Source: CAD feature listing. Evaluate the final solid. Frame: model axes, mm. Give positions to 0.01 mm unless a question says otherwise; leave off trailing zeros. Loops run counter-clockwise (first coordinate to the right, second up) from the corner with the lowest first, then second, coordinate; pieces in that order, holes last. Notation, with made-up numbers: (-27, 24.5) -> (-19, 24.5) arc R21 cw to (-19, 60.5) -> close; hole circle Ø10 at (37, 25.25). An arc over 180 degrees is marked (long way). Return JSON: item names as keys, results as strings. Group by question number.
(1) Ray query, line 1 (X direction, y = 2.6, z = -51.5); line 2 (Z direction, x = 35.75, y = 1.15) (3 decimals); line 3 (Z direction, x = -70.17, y = 1.1). Return the intervals inside material, ascending. Write a range as from..to.
(2) Cut plane B-B on x = -23. Return loops of the section in (y, z), then the cut area to 3 significant figures.
(3) Pin query (flat end, axial travel): pin 1 (2.5 mm diameter, centred on x = 82.67, z = -74.19, fed in from +Y). Return the tip coordinate at first contact, or that it passes through.
(4) Cut plane C-C on y = 2.4. Give the number of separate pieces and of enclosed holes in the cut face, then the cut area to 3 significant figures.
(5) Cut plane A-A on z = 33. Return loops of the section in (x, y), then the cut area to 3 significant figures.
```python
from build123d import *

# Parameters (mm, degrees)
SCHIZZO1_W                   = 180.34
SCHIZZO1_H                   = 227.22
ESTRUSIONE_ESTRUSIONE1_DEPTH = 3
SCHIZZO2_R                   = 1.5
SCHIZZO2_R_2                 = 3.25
SCHIZZO2_W                   = 5
SCHIZZO2_H                   = 18
TAGLIO_ESTRUSIONE1_DEPTH     = 4
SCHIZZO3_R                   = 1.5
TAGLIO_ESTRUSIONE5_DEPTH     = 4


with BuildPart() as part:
    # Schizzo1 → Estrusione-Estrusione1 (new body)
    with BuildSketch(Plane(origin=(0, 0, 0), x_dir=(1, 0, 0), z_dir=(0, 1, 0))):
        Rectangle(SCHIZZO1_W, SCHIZZO1_H)
    extrude(amount=ESTRUSIONE_ESTRUSIONE1_DEPTH)

    # Schizzo2 → Taglio-Estrusione1 (cut, through all)
    with BuildSketch(Plane(origin=(0, 0, 0), x_dir=(1, 0, 0), z_dir=(0, 1, 0))):
        with Locations((-82.67, -5.81)):
            Circle(SCHIZZO2_R)
        with Locations((-82.67, -87.31)):
            Circle(SCHIZZO2_R)
        with Locations((-82.67, 74.19)):
            Circle(SCHIZZO2_R)
        with Locations((82.67, -87.31)):
            Circle(SCHIZZO2_R)
        with Locations((82.67, -5.81)):
            Circle(SCHIZZO2_R)
        with Locations((82.67, 74.19)):
            Circle(SCHIZZO2_R)
        with Locations((-70.17, -78.61)):
            Circle(SCHIZZO2_R_2)
        with Locations((70.17, -78.61)):
            Circle(SCHIZZO2_R_2)
        with Locations((-30, 89.61)):
            Circle(SCHIZZO2_R)
        with Locations((-30, 108.61)):
            Circle(SCHIZZO2_R)
        with Locations((30, 89.61)):
            Circle(SCHIZZO2_R)
        with Locations((30, 108.61)):
            Circle(SCHIZZO2_R)
        with Locations((82.67, -49.13)):
            Rectangle(SCHIZZO2_W, SCHIZZO2_H)
        with Locations((-82.67, -49.13)):
            Rectangle(SCHIZZO2_W, SCHIZZO2_H)
        with Locations((-82.67, 47.19)):
            Rectangle(SCHIZZO2_W, SCHIZZO2_H)
        with Locations((82.67, 47.19)):
            Rectangle(SCHIZZO2_W, SCHIZZO2_H)
    extrude(amount=TAGLIO_ESTRUSIONE1_DEPTH, mode=Mode.SUBTRACT)

    # Schizzo3 → Taglio-Estrusione5 (cut, through all)
    with BuildSketch(Plane(origin=(0, 0, 0), x_dir=(1, 0, 0), z_dir=(0, 1, 0))):
        with Locations((-35.75, -77.045)):
            Circle(SCHIZZO3_R)
        with Locations((35.75, -77.045)):
            Circle(SCHIZZO3_R)
        with Locations((-35.75, 16.055)):
            Circle(SCHIZZO3_R)
        with Locations((35.75, 16.055)):
            Circle(SCHIZZO3_R)
        with BuildLine():
            Line((-31.5, -84.26), (-31.5, 23.27))
            ThreePointArc((-31.5, 23.27), (-30.225914498, 26.345914498), (-27.15, 27.62))
            Line((-27.15, 27.62), (27.15, 27.62))
            ThreePointArc((27.15, 27.62), (30.225914498, 26.345914498), (31.5, 23.27))
            Line((31.5, 23.27), (31.5, -84.26))
            ThreePointArc((31.5, -84.26), (30.225914498, -87.335914498), (27.15, -88.61))
            Line((27.15, -88.61), (-27.15, -88.61))
            ThreePointArc((-27.15, -88.61), (-30.225914498, -87.335914498), (-31.5, -84.26))
        make_face()
    extrude(amount=TAGLIO_ESTRUSIONE5_DEPTH, mode=Mode.SUBTRACT)


solid = part.part
```
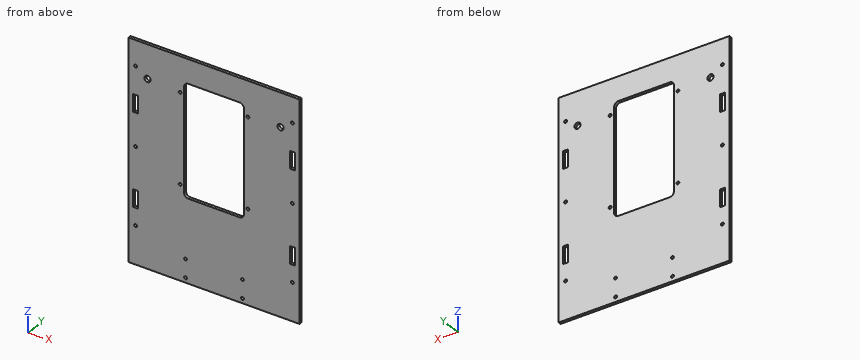
Answers:
{
 "1": {"line 1": "-90.17..-85.17, -80.17..80.17, 85.17..90.17", "line 2": "-113.61..-17.555, -14.555..75.545, 78.545..113.61", "line 3": "-113.61..75.36, 81.86..113.61"},
 "2": {"outline": "(0, -113.61) -> (3, -113.61) -> (3, -27.62) -> (0, -27.62) -> close; (0, 88.61) -> (3, 88.61) -> (3, 113.61) -> (0, 113.61) -> close", "area": "333 mm²"},
 "3": {"pin 1": "through"},
 "4": {"separate pieces": "1", "enclosed holes": "21", "area": "33,100 mm²"},
 "5": {"outline": "(-90.17, 0) -> (-31.5, 0) -> (-31.5, 3) -> (-90.17, 3) -> close; (31.5, 0) -> (90.17, 0) -> (90.17, 3) -> (31.5, 3) -> close", "area": "352 mm²"}
}
